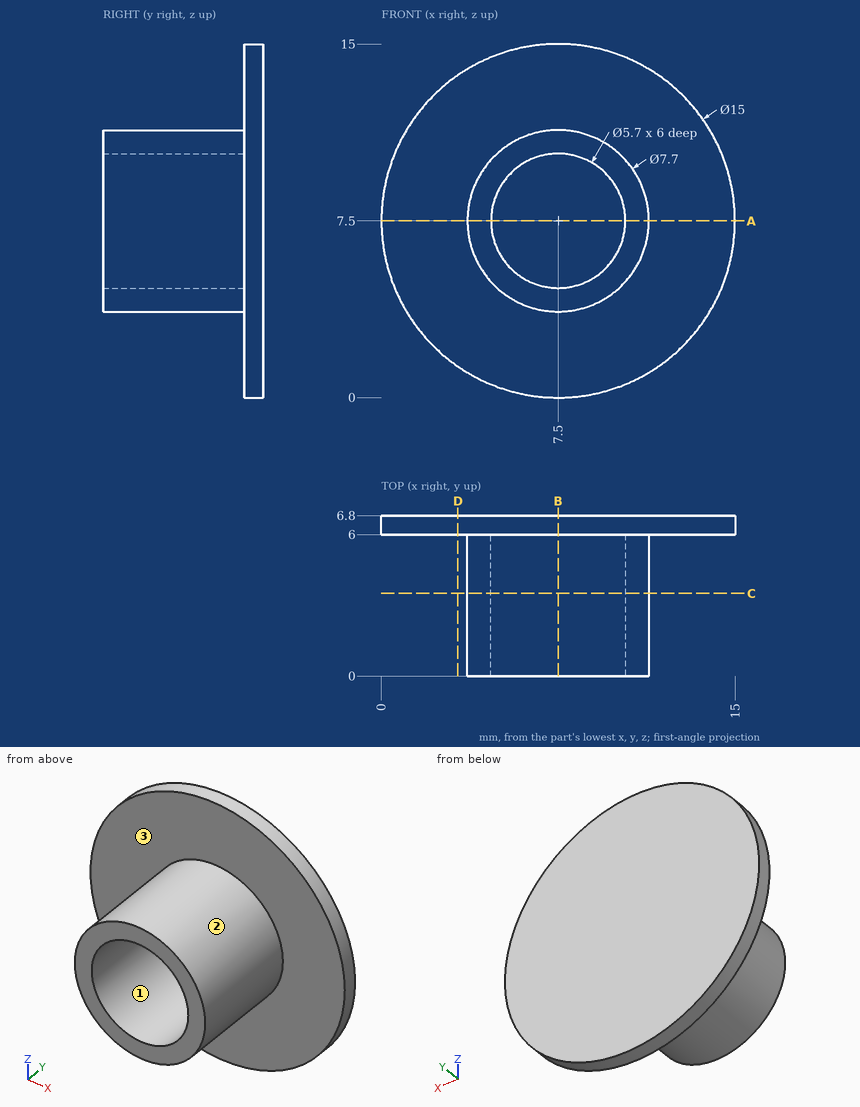
Could you check a few things on this drawing? It's one solid part, dimensions in mm from its lowest x, y, z. Give positions to 0.01 mm unless a question says otherwise; leave off trailing zeros. Write each loop counter-clockwise with the first axis right and the second up, starting at its lowest first coordinate (ties: lowest second). Pieces come first, ordered by that corner, then holes. Notation, with made-up numbers: (17, 20.5) -> (28, 20.5) arc R17 ccw to (28, 28.5) -> close; hole circle Ø2 at (22.25, -4.75). An arc over 180 degrees is marked (long way). Answer as a JSON object with one key per item and string values.
Q1. Suppose I cut it at B-B on x = 7.5. Write out the boundary of the cut face in (y, z), then the cut area to 3 significant figures.
Taken from the geometry:
{"outline": "(0, 3.65) -> (6, 3.65) -> (6, 0) -> (6.8, 0) -> (6.8, 15) -> (6, 15) -> (6, 11.35) -> (0, 11.35) -> (0, 10.35) -> (6, 10.35) -> (6, 4.65) -> (0, 4.65) -> close", "area": "24.0 mm²"}
Q2. Please list where these lines run through material, in increasing order: L1, parallel to Z at x = 7.5, y = 3.85; L2, parallel to Y at x = 13, z = 4.25; L3, parallel to X at y = 0.75, z = 8.75.
Taken from the geometry:
{"L1": "z = 3.65 to 4.65, 10.35 to 11.35", "L2": "y = 6 to 6.8", "L3": "x = 3.86 to 4.94, 10.06 to 11.14"}
Q3. Suppose I cut it at A-A on z = 7.5. Write out the boundary of the cut face in (x, y), then the cut area to 3 significant figures.
Taken from the geometry:
{"outline": "(0, 6) -> (3.65, 6) -> (3.65, 0) -> (4.65, 0) -> (4.65, 6) -> (10.35, 6) -> (10.35, 0) -> (11.35, 0) -> (11.35, 6) -> (15, 6) -> (15, 6.8) -> (0, 6.8) -> close", "area": "24.0 mm²"}
Q4. Suppose I cut it at C-C on y = 3.5. Write out the boundary of the cut face in (x, z).
Taken from the geometry:
{"outline": "circle Ø7.7 at (7.5, 7.5); hole circle Ø5.7 at (7.5, 7.5)"}
Q5. Suppose I cut it at D-D on x = 3.25. Write out the boundary of the cut face in (y, z).
Taken from the geometry:
{"outline": "(6, 1.32) -> (6.8, 1.32) -> (6.8, 13.68) -> (6, 13.68) -> close"}
Q6. We'd pull the mould along X, two halves only. Please class the marked faces 1, 2 and 3: released by +X, released by -X, zero draft, split by the parting line, or undercut.
Taken from the geometry:
{"face 1": "undercut", "face 2": "split by the parting line", "face 3": "zero draft"}
Q7. Will these pins go through, and if not, where does the flat tip stop? pin 1 Ø3 at (x, y) = (11, 5) entering from -Z; pin 2 Ø3 at (x, z) = (7.5, 8.5) entering from -Y; pin 3 Ø2 at (x, y) = (8.5, 3.5) entering from +Z.
Taken from the geometry:
{"pin 1": "stops at z = 0.39", "pin 2": "stops at y = 6", "pin 3": "stops at z = 11.35"}
